Autodesk Inventor part; units mm, degrees
ref_plane "YZ Plane" through (0, 0, 0) normal (1, 0, 0) x (0, 1, 0)
ref_plane "XZ Plane" through (0, 0, 0) normal (0, 1, 0) x (-1, 0, 0)
ref_plane "XY Plane" through (0, 0, 0) normal (0, 0, 1) x (1, 0, 0)
sketch "Profile Sketch" plane through (0, 0, 0) normal (1, 0, 0) x (0, 1, 0)
  line L0 (-2, 2.1422) -> (-2, 54.9636)
  arc A0 (11.247, 53.8378) -> (-2, 54.9636) centre (0, 0) ccw
  line L1 (13.6019, 50.4669) -> (6.1877, -0.2171)
  line L2 (-2, 2.1422) -> (0.3454, 0.4906)
  arc A1 (0, -0.6) -> (0.3454, 0.4906) centre (0, 0) ccw
  line L3 (0, -0.6) -> (-2, -0.6)
  line L4 (-2, -0.6) -> (-2, -8.1183)
  line L5 (-2, -8.1183) -> (-4.7049, -10.8232)
  line L6 (-4.7781, -11.25) -> (-2, -11.25)
  line L7 (4.7035, -1.5) -> (1.4679, -1.5)
  line L8 (1, -1.5) -> (2, -7)
  line L9 (2, -7) -> (-2, -11.25)
  line L10 (-2, 4.4659) -> (1.4394, 2.0441)
  arc A2 (2.3633, -0.8155) -> (1.4394, 2.0441) centre (0, 0) ccw
  line L11 (2.3633, -0.8155) -> (-0.027, -0.6)
  arc A3 (4.7035, -1.5) -> (6.1877, -0.2171) centre (4.7035, 0) ccw
  arc A4 (13.6019, 50.4669) -> (11.247, 53.8378) centre (10.6335, 50.9012) ccw
  line L12 (4.7035, 0) -> (0, 0) construction
  line L13 (1.4679, -1.5) -> (-2, -1.5)
  arc A5 (-4.7049, -10.8232) -> (-4.5281, -11.25) centre (-4.5281, -11) ccw
  line L14 (-4.7781, -11.25) -> (-4.7781, -11) construction
  point P0 (14, 53.1883)
  point P1 (6, -1.5)
  dimension "d0" = 0.6
  dimension "d2" = 45
  dimension "d4" = 55
  dimension "d7" = 54.848
  dimension "d8" = 2.5
  dimension "d9" = 5.152
  dimension "d10" = 2
  dimension "d11" = 16
  dimension "d12" = 8
  dimension "d13" = 1.5
  dimension "d14" = 3
  dimension "d20" = 2.7781
  dimension "d26" = 11
  dimension "d27" = 0.25
  dimension "d28" = 7
  dimension "d30" = 1
  dimension "d31" = 3
extrude "Main Key" add sketch "Profile Sketch" along normal mid plane 10.275 contours L0 L10 A2 L11 L3 A1 L2 | L0 A0 A4 L1 A3 L7 L13 L4 L3 L11 A2 L10
extrude "Extrusion2" add sketch "Profile Sketch" along normal mid plane 8 contours L13 L8 L9 L6 A5 L5 L4
fillet "Fillet1" radius 0.7 10 edges at (-5.1375, 5.6844, -1.1348) (-5.1375, 1.3517, -1.5) (-5.1375, 13.0928, 52.6193) (-5.1375, 4.6576, 54.8024) (-5.1375, 9.8948, 25.1249) (5.1375, 13.0928, 52.6193) (5.1375, 4.6576, 54.8024) (5.1375, 5.6844, -1.1348) (5.1375, 1.3517, -1.5) (5.1375, 9.8948, 25.1249)
extrude "Extrusion3" cut sketch "Profile Sketch" along normal mid plane 4.31 contours L0 L10 A2 L11 L3 A1 L2
fillet "Fillet2" radius 5 2 edges at (0, -2, -8.1183) (0, -2, -11.25)
fillet "Fillet3" radius 0.7 1 edges at (0, 2, -7)
equation "\"d0\" = hingeSocketRad"
equation "\"d4\" = blackKeyLength"
properties part number "black_key" material "PLA (Black, 3D Printed)"
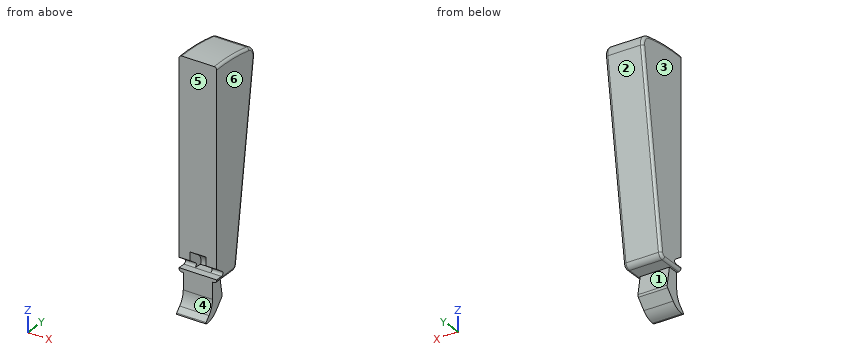
CAD build for the part. Positions are in the model's coordinates, mm. Face numbers are marked on the shaded views. A direction names the side the tool comes from. Give positions to 0.01 mm unless a question says otherwise; leave off trailing zeros. Write each loop counter-clockwise with the first axis right and the second up, starting at its lowest first coordinate (ties: lowest second). Pieces come first, ordered by that corner, then holes. Notation, with made-up numbers: (86.5, 67) -> (123.5, 67) arc R21 ccw to (123.5, 105) -> close; hole circle Ø9 at (85.5, 9). An arc over 180 degrees is marked (long way). Return JSON: item names as keys, results as strings.
Item 1: Drop flat-ended pins along their axis: pin 1 (2 mm diameter, centred on x = 2.5, y = 4.5, fed in from +Z); pin 2 (1.5 mm diameter, centred on x = 1.5, y = 1, fed in from +Z); pin 3 (6 mm diameter, centred on x = 1, z = -3.5, fed in from -Y). Give the stop position or say it passes through.
Answer below:
{"pin 1": "stops at z = 54.89", "pin 2": "stops at z = 55", "pin 3": "stops at y = -2.02"}
Item 2: Tool access for the marked faces 5 and 6: list every direction of +Z, -Z, +X, -X, +Y, -Y with a clear straight run to the whole face (end or side of a thin tool).
Answer below:
{"face 5": "+Z, +X, -X, -Y", "face 6": "+Z, -Z, +X, +Y, -Y"}
Item 3: Drill centre lines: probe 1 along Z at (x, y) = (2, -0.5); probe 2 along Y at (x, z) = (-0.5, 50.5); probe 3 along X at (y, z) = (0, -5.5). Where is each one in solid material? Low to high.
Answer below:
{"probe 1": "z = -9.66 to -0.6, 3.41 to 55", "probe 2": "y = -2 to 13.61", "probe 3": "x = -4 to 4"}
Item 4: Band-saw the part on A-A (x = -0.25). List the corners of the cut face in (y, z), then the cut area to 3 significant figures.
Answer below:
{"outline": "(-4.7, -10.82) arc R0.25 ccw to (-4.53, -11.25) -> (-4.16, -11.25) arc R5 ccw to (-0.52, -9.68) -> (1.76, -7.26) arc R0.7 ccw to (1.94, -6.65) -> (1, -1.5) -> (4.7, -1.5) arc R1.5 ccw to (6.19, -0.22) -> (13.6, 50.47) arc R3 ccw to (11.25, 53.84) arc R55 ccw to (-2, 54.96) -> (-2, 4.47) -> (1.44, 2.04) arc R2.5 cw to (2.36, -0.82) -> (-0.03, -0.6) -> (-2, -0.6) -> (-2, -6.05) arc R5 cw to (-3.46, -9.58) -> close", "area": "692 mm2"}
Item 5: Two-plate mould, pull along Z, no slides. Class the marked faces 1, 2, 3 and 4: +Z half, -Z half, draft (parallel to the pull), parting line (faces both ways), or undercut.
Answer below:
{"face 1": "undercut", "face 2": "-Z half", "face 3": "draft", "face 4": "+Z half"}
Item 6: Band-saw the part on B-B (z = -4). List the corners of the cut face in (x, y).
Answer below:
{"outline": "(-4, -2) -> (4, -2) -> (4, 1.45) -> (-4, 1.45) -> close"}
